For this review, take the finished solid that the model builds, in its own axes (mm). Give positions to 0.01 mm unless a question says otherwise; leave off trailing zeros. Loops run counter-clockwise (first coordinate to the right, second up) from the corner with the lowest first, then second, coordinate; pieces in that order, holes last.
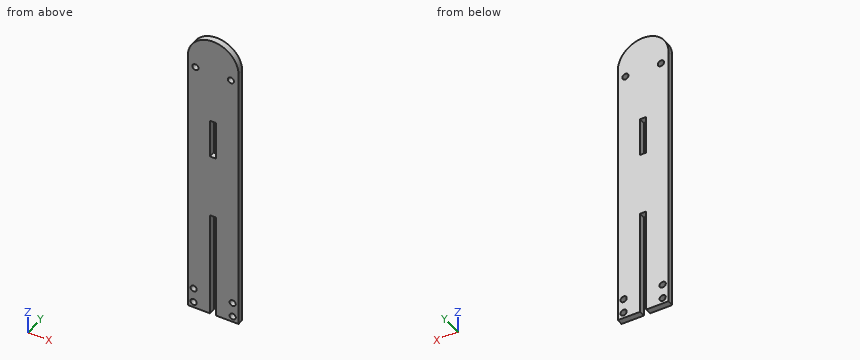
```python
from build123d import *

# Parameters (mm, degrees)
SKETCH1_W               = 3.175
SKETCH1_H               = 20
BOSS_EXTRUDE1_DEPTH     = 3.175
CUT_EXTRUDE2_DEPTH      = 154.72662678
CUT_EXTRUDE2_DEPTH_BACK = 154.72662678
SKETCH4_R               = 1.6
CUT_EXTRUDE3_DEPTH      = 154.72662678
CUT_EXTRUDE3_DEPTH_BACK = 154.72662678
SKETCH5_R               = 1.6


with BuildPart() as part:
    # Sketch1 → Boss-Extrude1 (new body)
    with BuildSketch(Plane(origin=(0, 0, 0), x_dir=(1, 0, 0), z_dir=(0, 1, 0))):
        with BuildLine():
            Line((-14.5875, 0), (-14.5875, -140))
            ThreePointArc((-14.5875, -140), (-1.5875, -153), (11.4125, -140))
            Line((11.4125, -140), (11.4125, 0))
            Line((11.4125, 0), (0, 0))
            Line((0, 0), (0, -55))
            Line((0, -55), (-3.175, -55))
            Line((-3.175, -55), (-3.175, 0))
            Line((-3.175, 0), (-14.5875, 0))
        make_face()
        with Locations((-1.5875, -98)):
            Rectangle(SKETCH1_W, SKETCH1_H, mode=Mode.SUBTRACT)
    extrude(amount=BOSS_EXTRUDE1_DEPTH)

    # Sketch4 → Cut-Extrude2 (cut, two sides: drawn at the far end of the back side and taken through both)
    with BuildSketch(Plane.XZ.offset(-CUT_EXTRUDE2_DEPTH_BACK)):
        with Locations(Location((8.4125, 3, 0), (0, 0, 270))):
            Circle(SKETCH4_R)
        with Locations(Location((8.4125, 10.5, 0), (0, 0, 270))):
            Circle(SKETCH4_R)
        with Locations(Location((-11.5875, 10.5, 0), (0, 0, 270))):
            Circle(SKETCH4_R)
        with Locations(Location((-11.5875, 3, 0), (0, 0, 270))):
            Circle(SKETCH4_R)
    extrude(amount=CUT_EXTRUDE2_DEPTH + CUT_EXTRUDE2_DEPTH_BACK, mode=Mode.SUBTRACT)

    # Sketch5 → Cut-Extrude3 (cut, two sides: drawn at the far end of the back side and taken through both)
    with BuildSketch(Plane(origin=(0, 3.175, 0), x_dir=(1, 0, 0), z_dir=(0, 1, 0)).offset(-CUT_EXTRUDE3_DEPTH_BACK)):
        with Locations(Location((-10.675, -135, 0), (0, 0, 270))):
            Circle(SKETCH5_R)
        with Locations(Location((7.5, -135, 0), (0, 0, 270))):
            Circle(SKETCH5_R)
    extrude(amount=CUT_EXTRUDE3_DEPTH + CUT_EXTRUDE3_DEPTH_BACK, mode=Mode.SUBTRACT)


solid = part.part
```
Item 1: For L1, parallel to X at y = 2.3, z = 3 (1 decimal); L2, parallel to X at y = 0.7, z = 135 (1 decimal); L3, parallel to X at y = 0.55, z = 53.5 (1 decimal), list the stretches that pass through material, from the lowest coordinate up.
Answer:
L1: x = -14.6 to -13.2, -10 to -3.2, 0 to 6.8, 10 to 11.4
L2: x = -14.6 to -12.3, -9.1 to 5.9, 9.1 to 11.4
L3: x = -14.6 to -3.2, 0 to 11.4
Item 2: Take a section at A-A on z = 135. Give the boundary of the cut face in (x, y) (1 decimal).
Answer:
outline: (-14.6, 0) - (-12.3, 0) - (-12.3, 3.2) - (-14.6, 3.2) - close; (-9.1, 0) - (5.9, 0) - (5.9, 3.2) - (-9.1, 3.2) - close; (9.1, 0) - (11.4, 0) - (11.4, 3.2) - (9.1, 3.2) - close
Item 3: Take a section at D-D on y = 1.45. Give the boundary of the cut face in (x, z) (1 decimal).
Answer:
outline: (-14.6, 0) - (-3.2, 0) - (-3.2, 55) - (0, 55) - (0, 0) - (11.4, 0) - (11.4, 140) arc R13 ccw to (-14.6, 140) - close; hole circle Ø3.2 at (-11.6, 3); hole circle Ø3.2 at (-11.6, 10.5); hole circle Ø3.2 at (-10.7, 135); hole (-3.2, 88) - (0, 88) - (0, 108) - (-3.2, 108) - close; hole circle Ø3.2 at (7.5, 135); hole circle Ø3.2 at (8.4, 3); hole circle Ø3.2 at (8.4, 10.5)
Item 4: Take a section at B-B on z = 37. Give the boundary of the cut face in (x, y) (1 decimal), and give its area (3 significant figures).
Answer:
outline: (-14.6, 0) - (-3.2, 0) - (-3.2, 3.2) - (-14.6, 3.2) - close; (0, 0) - (11.4, 0) - (11.4, 3.2) - (0, 3.2) - close
area: 72.5 mm2
Item 5: Take a section at C-C on z = 3. Give the boundary of the cut face in (x, y) (1 decimal).
Answer:
outline: (-14.6, 0) - (-13.2, 0) - (-13.2, 3.2) - (-14.6, 3.2) - close; (-10, 0) - (-3.2, 0) - (-3.2, 3.2) - (-10, 3.2) - close; (0, 0) - (6.8, 0) - (6.8, 3.2) - (0, 3.2) - close; (10, 0) - (11.4, 0) - (11.4, 3.2) - (10, 3.2) - close
